Source: three-view drawing plus pictorial views. Frame: mm from the lowest corner of the part. Give positions to 0.01 mm unless a question says otherwise; leave off trailing zeros. Loops run counter-clockwise (first coordinate to the right, second up) from the corner with the lowest first, then second, coordinate; pieces in that order, holes last. Notation, with made-up numbers: M 20.5,-11 L 75.5,-11 A24 ccw 75.5,-1 Z; hole C 31.5,86.25 d11. An arc over 180 degrees is marked long. Answer as a JSON object with one key per item and string values. Group by question number.
1) Section query A-A on x = 12. Return loops of the section in (y, z), plus the area to 3 significant figures.
2) Ray query, L1, parallel to X at y = 82.5, z = 0.1; L2, parallel to Y at x = 12, z = 2.3; L3, parallel to X at y = 26, z = 2.35. Return the intervals inside material, ascending.
3) Section query D-D on z = 0.8. Count the separate pieces of the cut face and the enclosed holes in it, plus the area to 3 significant figures.
4) First-contact query: P1, Ø1.5, axis at y = 97, z = 1.5, coming from the -X side; P2, Ø0.9, axis at y = 5.5, z = 1.5, coming from the +X side. Flat tips, straight axial feed; report the tip coordinate or a pass-through.
5) Section query B-B on y = 22. Return loops of the section in (x, z).
6) Section query C-C on x = 25.5. Return loops of the section in (y, z).
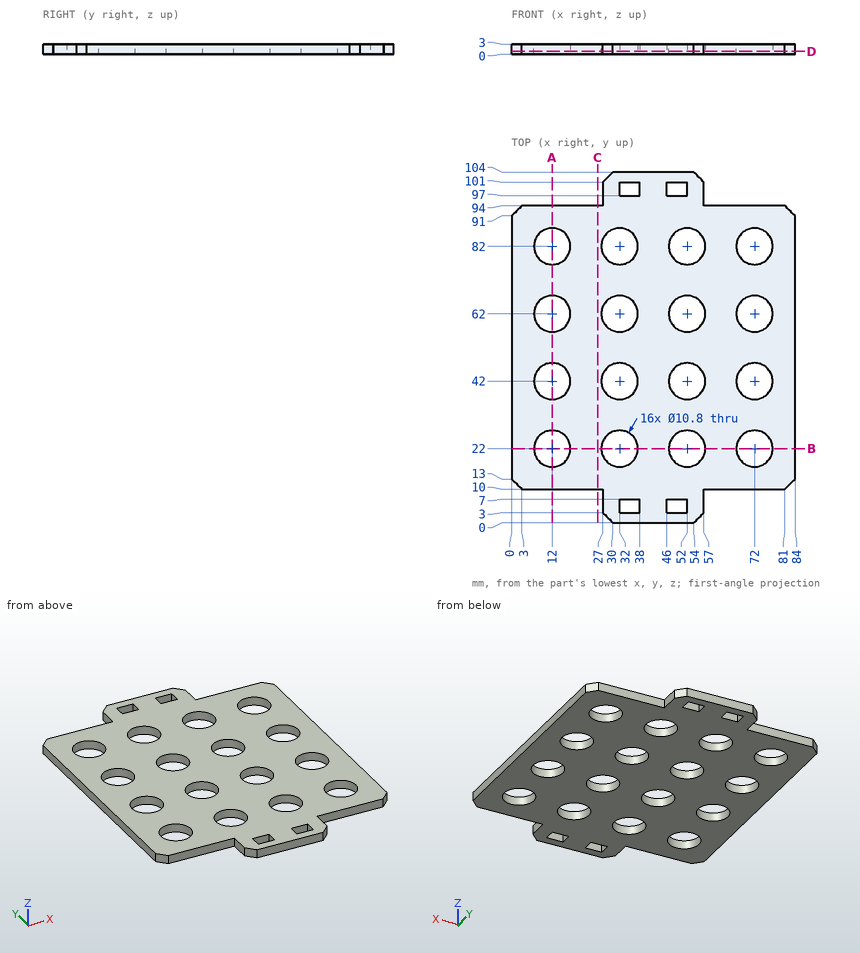
Output:
{
 "1": {"outline": "M 10,0 L 16.6,0 L 16.6,3 L 10,3 Z; M 27.4,0 L 36.6,0 L 36.6,3 L 27.4,3 Z; M 47.4,0 L 56.6,0 L 56.6,3 L 47.4,3 Z; M 67.4,0 L 76.6,0 L 76.6,3 L 67.4,3 Z; M 87.4,0 L 94,0 L 94,3 L 87.4,3 Z", "area": "122 mm^2"},
 "2": {"L1": "x = 0 to 6.62, 17.38 to 26.62, 37.38 to 46.62, 57.38 to 66.62, 77.38 to 84", "L2": "y = 10 to 16.6, 27.4 to 36.6, 47.4 to 56.6, 67.4 to 76.6, 87.4 to 94", "L3": "x = 0 to 8.37, 15.63 to 28.37, 35.63 to 48.37, 55.63 to 68.37, 75.63 to 84"},
 "3": {"separate pieces": "1", "enclosed holes": "20", "area": "6,060 mm^2"},
 "4": {"P1": "stops at x = 27", "P2": "stops at x = 57"},
 "5": {"outline": "M 0,0 L 6.6,0 L 6.6,3 L 0,3 Z; M 17.4,0 L 26.6,0 L 26.6,3 L 17.4,3 Z; M 37.4,0 L 46.6,0 L 46.6,3 L 37.4,3 Z; M 57.4,0 L 66.6,0 L 66.6,3 L 57.4,3 Z; M 77.4,0 L 84,0 L 84,3 L 77.4,3 Z"},
 "6": {"outline": "M 10,0 L 94,0 L 94,3 L 10,3 Z"}
}
